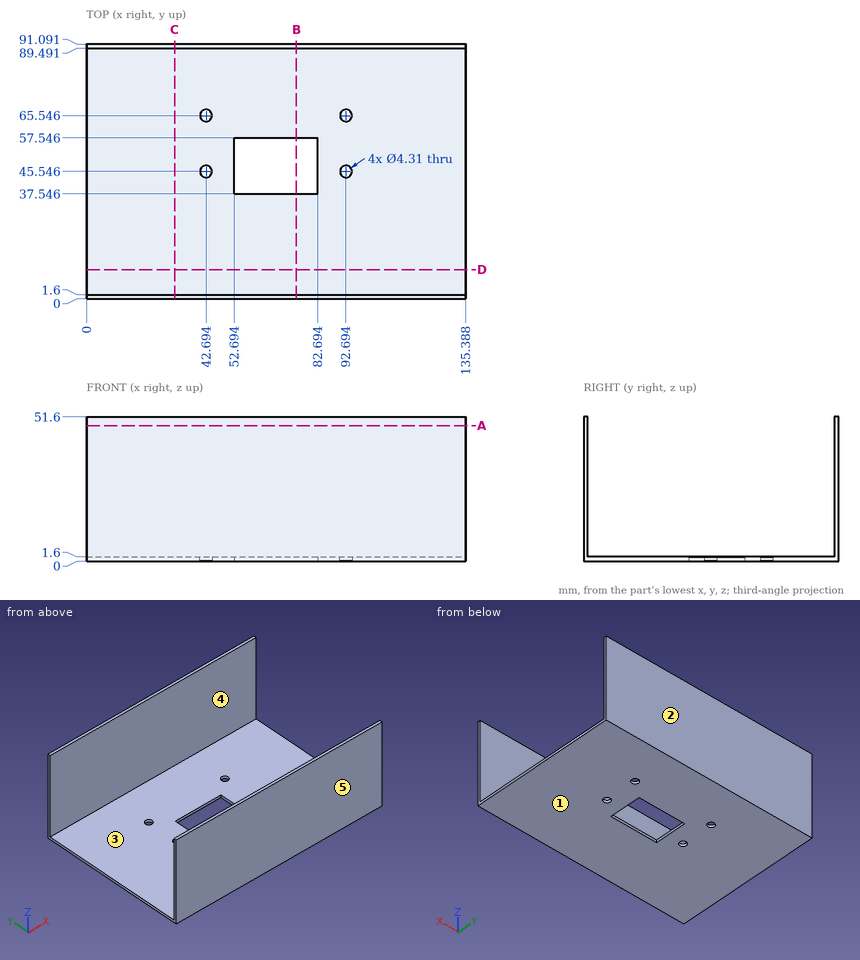
Could you check a few things on this drawing? It's one solid part, dimensions in mm from its lowest x, y, z. A direction names the side the tool comes from. Round coordinates to 2 decimals unless told otherwise and drop trailing zeros. Order: outer loops, then holes, each group sorted by start corner. A loop starts at its lowest first (then second) coordinate and runs counter-clockwise, first axis right, second up. Notation, with made-up numbers: M 82,22 L 134,22 A23 ccw 134,44 Z; hole C -39.5,22.25 d9. An arc over 180 degrees is marked long. One line per question, with ' | ' between items. Start each with the question number.
(1) Suppose I cut it at A-A on z = 48.5. List the corners of the cut face in (x, y) for me.
(2) For P1, Ø1, axis at x = 39, y = 33, coming from the +Z side; P2, Ø2.5, axis at x = 42.69, y = 45.55, coming from the +Z side, each with a flat end and sliding along its axis, tell me the tip position at first contact or that it passes through.
(3) For the marked faces 4 and 5, which set-ups out of +Z, -Z, +X, -X, +Y, -Y let a thin tool reach every point of the face, with its end or its side?
(4) Suppose I cut it at D-D on y = 10.5. List the corners of the cut face in (x, z) for me.
(5) Suppose I cut it at B-B on x = 75. List the corners of the cut face in (y, z) for me (1 decimal).
(6) Please list where these lines run through material, in increasing order: line 1 along Y through (x, z) = (13.5, 10.5); line 2 along Z through (x, y) = (75.5, 21.5).
(7) Suppose I cut it at C-C on x = 31.5. List the corners of the cut face in (y, z) for me.
(8) Thinking about a two-plate mould opening in Y: for the marked faces 1, 2 and 3, which applies, +Y half, -Y half, draft (parallel to the pull), parting line (faces both ways), or undercut?
Geometry results:
1) outline: M 0,0 L 135.39,0 L 135.39,1.6 L 0,1.6 Z; M 0,89.49 L 135.39,89.49 L 135.39,91.09 L 0,91.09 Z
2) P1: z = 1.6 | P2: through
3) face 4: +Z, +X, -X | face 5: +Z, -Z, +X, -X, -Y
4) outline: M 0,0 L 135.39,0 L 135.39,1.6 L 0,1.6 Z
5) outline: M 0,0 L 37.5,0 L 37.5,1.6 L 1.6,1.6 L 1.6,51.6 L 0,51.6 Z; M 57.5,0 L 91.1,0 L 91.1,51.6 L 89.5,51.6 L 89.5,1.6 L 57.5,1.6 Z
6) line 1: 0 to 1.6, 89.49 to 91.09 | line 2: 0 to 1.6
7) outline: M 0,0 L 91.09,0 L 91.09,51.6 L 89.49,51.6 L 89.49,1.6 L 1.6,1.6 L 1.6,51.6 L 0,51.6 Z
8) face 1: draft | face 2: +Y half | face 3: undercut
